Design review of the part built by this model. Coordinates are the model's own, in mm. Face numbers are marked on the shaded views. A direction names the side the tool comes from. Round coordinates to 2 decimals unless told otherwise and drop trailing zeros. Order: outer loops, then holes, each group sorted by start corner. A loop starts at its lowest first (then second) coordinate and runs counter-clockwise, first axis right, second up. Notation, with made-up numbers: (58.25, -11) - (66.25, -11) arc R33 cw to (66.25, 26) - close; hole circle Ø3 at (67.25, -31.5). An arc over 180 degrees is marked (long way). Use CSV: the item, a comma, the result in double quotes.
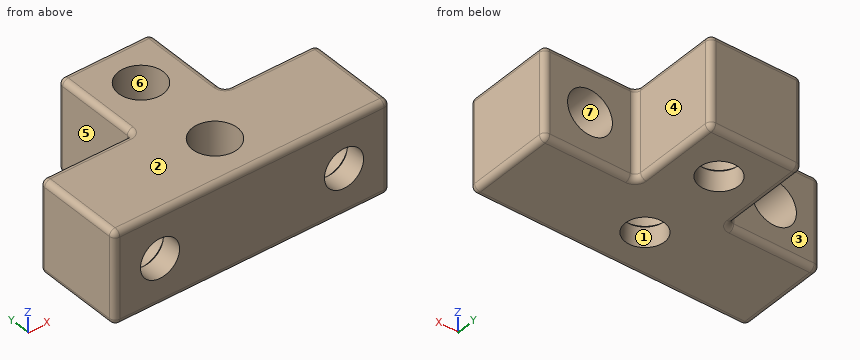
from build123d import *

# Parameters (mm, degrees)
BOSS_EXTRUDE1_DEPTH                      = 8
F_3_9_3_9_DIAMETER_HOLE1_D               = 3.9
F_3_9_3_9_DIAMETER_HOLE1_DEPTH           = 6
F_3_9_3_9_DIAMETER_HOLE1_TIP             = 1.95
F_3_9_3_9_DIAMETER_HOLE1_ON_FACE_2_D     = 3.9
F_3_9_3_9_DIAMETER_HOLE1_ON_FACE_2_DEPTH = 6
F_3_9_3_9_DIAMETER_HOLE1_ON_FACE_2_TIP   = 1.95
F_3_4_3_4_DIAMETER_HOLE1_OUTLINE_R       = 1.7
F_3_4_3_4_DIAMETER_HOLE1_DEPTH           = 1.7500001
F_3_4_3_4_DIAMETER_HOLE1_2_OUTLINE_R     = 1.7
F_3_4_3_4_DIAMETER_HOLE1_2_DEPTH         = 1.7500001
FILLET1_R                                = 0.5


# Read off the part's stored shape, not the designer's step: Ø3.4 (3.4) Diameter Hole1
with BuildPart() as part:
    # Sketch1 → Boss-Extrude1 (new body)
    with BuildSketch(Plane.XY):
        Polygon((-12, 0), (12, 0), (12, 8), (4, 8), (4, 16), (-4, 16), (-4, 8), (-12, 8), align=None)
    extrude(amount=BOSS_EXTRUDE1_DEPTH)

    # Ø3.9 (3.9) Diameter Hole1
    with Locations(Plane(origin=(0, 4, 8), x_dir=(1, 0, 0), z_dir=(0, 0, 1))):
        with Locations((0, 0), (0, 8)):
            Hole(F_3_9_3_9_DIAMETER_HOLE1_D / 2, depth=F_3_9_3_9_DIAMETER_HOLE1_DEPTH)
            with Locations((0, 0, -(F_3_9_3_9_DIAMETER_HOLE1_DEPTH + F_3_9_3_9_DIAMETER_HOLE1_TIP / 2))):  # 90° drill point
                Cone(0, F_3_9_3_9_DIAMETER_HOLE1_D / 2, F_3_9_3_9_DIAMETER_HOLE1_TIP, mode=Mode.SUBTRACT)

    # Ø3.9 (3.9) Diameter Hole1 on face 2
    with Locations(Plane(origin=(8, 8, 4), x_dir=(0, 0, 1), z_dir=(0, 1, 0))):
        with Locations((0, 0), (0, -16)):
            Hole(F_3_9_3_9_DIAMETER_HOLE1_ON_FACE_2_D / 2, depth=F_3_9_3_9_DIAMETER_HOLE1_ON_FACE_2_DEPTH)
            with Locations((0, 0, -(F_3_9_3_9_DIAMETER_HOLE1_ON_FACE_2_DEPTH + F_3_9_3_9_DIAMETER_HOLE1_ON_FACE_2_TIP / 2))):  # 90° drill point
                Cone(0, F_3_9_3_9_DIAMETER_HOLE1_ON_FACE_2_D / 2, F_3_9_3_9_DIAMETER_HOLE1_ON_FACE_2_TIP, mode=Mode.SUBTRACT)

    # Ø3.4 (3.4) Diameter Hole1 outline → Ø3.4 (3.4) Diameter Hole1 (cut)
    with BuildSketch(Plane(origin=(0, 0, 0), x_dir=(1, 0, 0), z_dir=(0, 1, 0))):
        with Locations((-8, -4)):
            Circle(F_3_4_3_4_DIAMETER_HOLE1_OUTLINE_R)
        with Locations((8, -4)):
            Circle(F_3_4_3_4_DIAMETER_HOLE1_OUTLINE_R)
    extrude(amount=F_3_4_3_4_DIAMETER_HOLE1_DEPTH, mode=Mode.SUBTRACT)

    # 3.4 _3.4_ Diameter Hole1 2 outline → 3.4 _3.4_ Diameter Hole1 2 (cut)
    with BuildSketch(Plane.XY):
        with Locations((0, 4)):
            Circle(F_3_4_3_4_DIAMETER_HOLE1_2_OUTLINE_R)
        with Locations((0, 12)):
            Circle(F_3_4_3_4_DIAMETER_HOLE1_2_OUTLINE_R)
    extrude(amount=F_3_4_3_4_DIAMETER_HOLE1_2_DEPTH, mode=Mode.SUBTRACT)

    # Fillet1
    fillet1_edges = [part.edges().sort_by_distance(p)[0] for p in [
        (8, 8, 0),
        (12, 4, 0),
        (0, 0, 0),
        (-12, 4, 0),
        (12, 4, 8),
        (-12, 8, 4),
        (-4, 8, 4),
        (-4, 16, 4),
        (4, 16, 4),
        (4, 8, 4),
        (12, 8, 4),
        (12, 0, 4),
        (-12, 0, 4),
        (8, 8, 8),
        (4, 12, 8),
        (0, 16, 8),
        (-4, 12, 8),
        (-8, 8, 8),
        (-12, 4, 8),
        (-8, 8, 0),
        (0, 0, 8),
        (-4, 12, 0),
        (0, 16, 0),
        (4, 12, 0),
    ]]
    fillet(fillet1_edges, radius=FILLET1_R)


solid = part.part
1) To check wall thickness, follow L1, parallel to X at y = 0.85, z = 4; L2, parallel to Z at x = 8, y = 5.5; L3, parallel to Y at x = -1, z = 6. State the ranges of each line that lie inside material, in increasing order. Write a range as from..to.
Data:
L1,"x = -12..-9.7, -6.3..6.3, 9.7..12"
L2,"z = 0..2.05, 5.95..8"
L3,"y = 0..2.33, 5.67..10.33, 13.67..16"
2) We need section D-D (x = 8). Give the boundary of the cut face in (y, z), then the cut area to 3 significant figures.
Data:
outline,"(0, 0.5) arc R0.5 ccw to (0.5, 0) - (7.5, 0) arc R0.5 ccw to (8, 0.5) - (8, 2.05) - (2, 2.05) - (1.75, 2.3) - (0, 2.3) - close; (0, 5.7) - (1.75, 5.7) - (2, 5.95) - (8, 5.95) - (8, 7.5) arc R0.5 ccw to (7.5, 8) - (0.5, 8) arc R0.5 ccw to (0, 7.5) - close"
area,"33.5 mm2"
3) We need section B-B (y = 4). Give the boundary of the cut face in (x, z).
Data:
outline,"(-12, 0.5) arc R0.5 ccw to (-11.5, 0) - (-1.7, 0) - (-1.7, 1.75) - (-1.95, 2) - (-1.95, 8) - (-11.5, 8) arc R0.5 ccw to (-12, 7.5) - close; (1.7, 0) - (11.5, 0) arc R0.5 ccw to (12, 0.5) - (12, 7.5) arc R0.5 ccw to (11.5, 8) - (1.95, 8) - (1.95, 2) - (1.7, 1.75) - close; hole circle Ø3.9 at (-8, 4); hole circle Ø3.9 at (8, 4)"
4) We need section A-A (x = 0). Give the boundary of the cut face in (y, z), then the cut area to 3 significant figures.
Data:
outline,"(0, 0.5) arc R0.5 ccw to (0.5, 0) - (2.3, 0) - (2.3, 1.75) - (2.05, 2) - (2.05, 8) - (0.5, 8) arc R0.5 ccw to (0, 7.5) - close; (5.7, 0) - (10.3, 0) - (10.3, 1.75) - (10.05, 2) - (10.05, 8) - (5.95, 8) - (5.95, 2) - (5.7, 1.75) - close; (13.7, 0) - (15.5, 0) arc R0.5 ccw to (16, 0.5) - (16, 7.5) arc R0.5 ccw to (15.5, 8) - (13.95, 8) - (13.95, 2) - (13.7, 1.75) - close"
area,"67.3 mm2"
5) The part is to be moulded in two halves that separate along Y. For the marked faces 1, 2 and 3, say which applies: +Y half, -Y half, draft (parallel to the pull), parting line (faces both ways), or undercut.
Data:
face 1,"undercut"
face 2,"draft"
face 3,"+Y half"
6) For the marked faces 4, 5, 6 and 7, list the 3-axis set-ups (+Z, -Z, +X, -X, +Y, -Y) from which the entire face can be reached by the end or side of a thin tool; tool diameter is ignored.
Data:
face 4,"+Z, -Z, +X, +Y"
face 5,"+Z, -Z, -X, +Y"
face 6,"+Z"
face 7,"+Y"
7) We need section C-C (z = 4). Give the number of separate pieces and of enclosed holes in the cut face, then the cut area to 3 significant figures.
Data:
separate pieces,"3"
enclosed holes,"2"
area,"171 mm2"
8) Insertion check: pin 1 Ø4 at (x, z) = (-8, 4) entering from +Y. The pin has a flat end and moves straight along its axis. Give the tip position at first contact, or say it passes through.
Data:
pin 1,"stops at y = 8"
